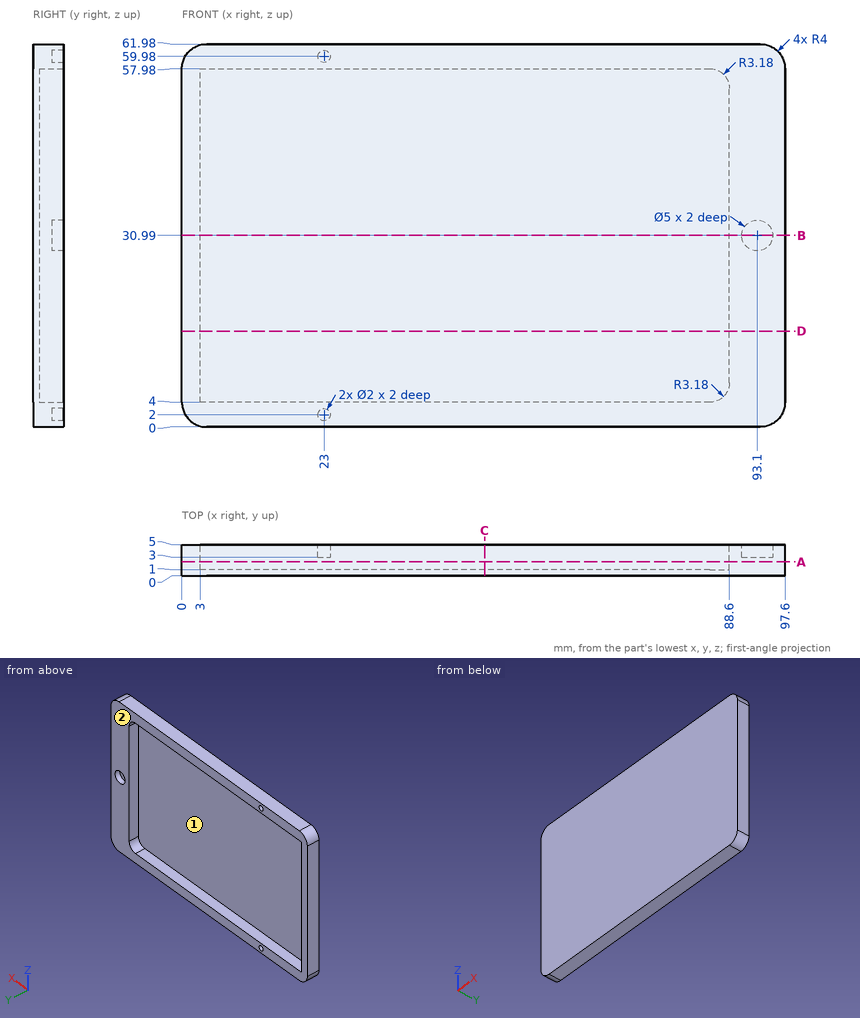
Geometry check sheet. Reference: drawing and pictorial views, mm from the part's lowest x, y, z. Coordinates: 2 decimals unless noted, no trailing zeros. Loops run counter-clockwise (first coordinate to the right, second up) from the corner with the lowest first, then second, coordinate; pieces in that order, holes last.
1) Sectioned sample at D-D (z = 15.5). Record the boundary of the cut face in (x, y).
2) Material ranges on probe 1 along Z at (x, y) = (23, 4.3); probe 2 along Z at (x, y) = (13, 4.25); probe 3 along X at (y, z) = (3.8, 51.5), recorded low to high.
3) Release check for a two-part mould opening along X. For the marked faces 1 and 2 record: released by +X, released by -X, zero draft, split by the parting line, or undercut.
4) Gauge pin test, flat ends, axial feed: pin 1 (2.5 mm diameter, centred on x = 23, z = 2, fed in from -Y); pin 2 (0.6 mm diameter, centred on x = 22.5, z = 2, fed in from +Y); pin 3 (6 mm diameter, centred on x = 19, z = 50.5, fed in from +Y). Record the tip position at first contact, or that the pin passes through.
5) Sectioned sample at A-A (y = 2.25). Record the boundary of the cut face in (x, z).
6) Sectioned sample at B-B (z = 30.99). Record the boundary of the cut face in (x, y), and give its area (3 significant figures).
7) Sectioned sample at C-C (x = 49). Record the boundary of the cut face in (y, z), and give its area (3 significant figures).
Check sheet entries:
1. outline: (0, 0) - (97.6, 0) - (97.6, 5) - (88.6, 5) - (88.6, 1) - (3, 1) - (3, 5) - (0, 5) - close
2. probe 1: z = 0 to 1, 3 to 4, 57.98 to 58.98, 60.98 to 61.98
2. probe 2: z = 0 to 4, 57.98 to 61.98
2. probe 3: x = 0 to 3, 88.6 to 97.6
3. face 1: undercut
3. face 2: zero draft
4. pin 1: stops at y = 0
4. pin 2: stops at y = 3
4. pin 3: stops at y = 1
5. outline: (0, 4) arc R4 ccw to (4, 0) - (93.6, 0) arc R4 ccw to (97.6, 4) - (97.6, 57.98) arc R4 ccw to (93.6, 61.98) - (4, 61.98) arc R4 ccw to (0, 57.98) - close; hole (3, 4) - (85.42, 4) arc R3.18 ccw to (88.6, 7.18) - (88.6, 54.8) arc R3.18 ccw to (85.42, 57.98) - (3, 57.98) - close
6. outline: (0, 0) - (97.6, 0) - (97.6, 5) - (95.6, 5) - (95.6, 3) - (90.6, 3) - (90.6, 5) - (88.6, 5) - (88.6, 1) - (3, 1) - (3, 5) - (0, 5) - close
6. area: 136 mm2
7. outline: (0, 0) - (5, 0) - (5, 4) - (1, 4) - (1, 57.98) - (5, 57.98) - (5, 61.98) - (0, 61.98) - close
7. area: 94.0 mm2
